```python
from build123d import *

# Parameters (mm, degrees)
ESBO_O1_R                = 2.5
RESSALTO_EXTRUS_O1_DEPTH = 245


with BuildPart() as part:
    # Esboço1 → Ressalto-extrusão1 (new, symmetric)
    with BuildSketch(Plane(origin=(0, 0, 0), x_dir=(0, 0, -1), z_dir=(1, 0, 0))):
        with BuildLine():
            Line((-200, -19.346040211), (-200, 35.835787631))
            Line((-200, 35.835787631), (-135.24, 35.835787631))
            ThreePointArc((-135.24, 35.835787631), (-66.489751819, 42.094735918), (0, 60.665787631))
            ThreePointArc((0, 60.665787631), (66.489751819, 42.094735918), (135.24, 35.835787631))
            Line((135.24, 35.835787631), (200, 35.835787631))
            Line((200, 35.835787631), (200, -15.024212369))
            ThreePointArc((200, -15.024212369), (203.164975379, -22.665138853), (195.524048894, -19.500163474))
            Line((195.524048894, -19.500163474), (186.500073192, -19.500163474))
            Line((186.500073192, -19.500163474), (85.729991436, -19.354819463))
            ThreePointArc((85.729991436, -19.354819463), (81.225610372, -23.84603807), (76.73, -19.346040211))
            Line((76.73, -19.346040211), (-200, -19.346040211))
        make_face()
        with Locations((81.23, -19.346040211)):
            Circle(ESBO_O1_R, mode=Mode.SUBTRACT)
        with Locations((200, -19.500163474)):
            Circle(ESBO_O1_R, mode=Mode.SUBTRACT)
    extrude(amount=RESSALTO_EXTRUS_O1_DEPTH, both=True)


solid = part.part
```
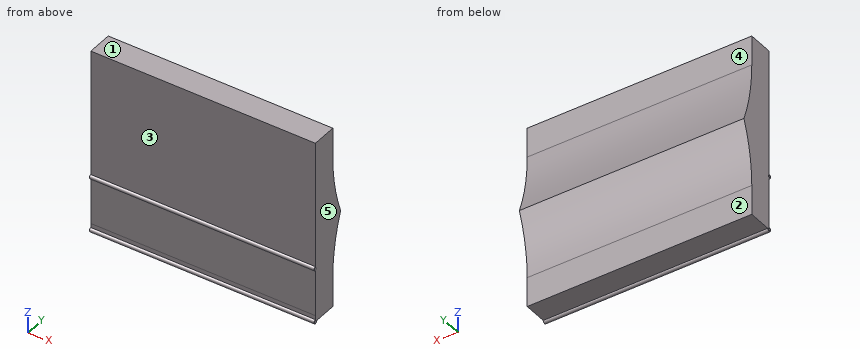
Check sheet for the modelled part. Datum: model origin and axes. Units: mm. Face numbers are marked on the shaded views. A direction names the side the tool comes from. Round coordinates to 2 decimals unless told otherwise and drop trailing zeros. Loops run counter-clockwise (first coordinate to the right, second up) from the corner with the lowest first, then second, coordinate; pieces in that order, holes last. Notation, with made-up numbers: (26, 13.25) -> (68, 13.25) arc R22 cw to (68, 28.25) -> close; hole circle Ø11 at (-26.75, 54.25). An arc over 180 degrees is marked (long way). Answer in a Markdown table with one row per item.
Q1. Sectioned sample at C-C on z = -42.5. Enter the section's corners in (x, y).
Data:
| item | result |
|---|---|
| outline | (-245, -19.35) -> (245, -19.35) -> (245, 47.3) -> (-245, 47.3) -> close |
Q2. Thickness scan on L1, parallel to Z at x = 85, y = -20; L2, parallel to Y at x = -194, z = -134.5; L3, parallel to Z at x = -146, y = -12. Record the ranges inside material, lowest first.
Data:
| item | result |
|---|---|
| L1 | z = -204.45 to -202.45, -197.55 to -195.55, -85.68 to -83.64, -78.82 to -76.78 |
| L2 | y = -19.43 to 35.84 |
| L3 | z = -200 to 200 |
Q3. Set-up check for the marked faces 1, 2, 3, 4 and 5: record each of +Z, -Z, +X, -X, +Y, -Y from which the full face is reachable in a straight line by a thin tool's end or side.
Data:
| item | result |
|---|---|
| face 1 | +Z, +X, -X, +Y, -Y |
| face 2 | -Z, +X, -X, +Y |
| face 3 | +Z, +X, -X, -Y |
| face 4 | +Z, +X, -X, +Y |
| face 5 | +Z, -Z, +X, +Y, -Y |
Q4. Sectioned sample at A-A on x = 206. Enter the section's corners in (y, z), then the cut area to 3 significant figures.
Data:
| item | result |
|---|---|
| outline | (-19.5, -195.52) arc R4.48 ccw (long way) to (-15.02, -200) -> (35.84, -200) -> (35.84, -135.24) arc R380.72 cw to (60.67, 0) arc R380.72 cw to (35.84, 135.24) -> (35.84, 200) -> (-19.35, 200) -> (-19.35, -76.73) arc R4.5 ccw to (-19.35, -85.73) -> (-19.5, -186.5) -> close; hole circle Ø5 at (-19.5, -200); hole circle Ø5 at (-19.35, -81.23) |
| area | 24,300 mm^2 |
Q5. Go/stop test with flat-tipped pins: P1, Ø8, axis at x = -72.5, y = 29.5, coming from the -Z side; P2, Ø3, axis at y = 37, z = -125, coming from the -X side; P3, Ø8, axis at x = -139.5, z = -32.5, coming from the +Y side; P4, Ø2, axis at x = 54, z = -94, coming from the -Y side. Record where each tip stops, or that it passes through.
Data:
| item | result |
|---|---|
| P1 | stops at z = -200 |
| P2 | stops at x = -245 |
| P3 | stops at y = 51.11 |
| P4 | stops at y = -19.37 |
Q6. Sectioned sample at B-B on z = -104. Enter the section's corners in (x, y).
Data:
| item | result |
|---|---|
| outline | (-245, -19.38) -> (245, -19.38) -> (245, 37.12) -> (-245, 37.12) -> close |
